For this review, use the dimensioned drawing (mm, ordinates from the lowest corner) and the shaded views. A direction names the side the tool comes from. Coordinates: 2 decimals unless noted, no trailing zeros. Loops run counter-clockwise (first coordinate to the right, second up) from the corner with the lowest first, then second, coordinate; pieces in that order, holes last. Notation, with made-up numbers: (-32, 59) -> (3, 59) arc R17 cw to (3, 75) -> close; hole circle Ø1 at (-6, 47.25). An arc over 180 degrees is marked (long way). Answer as a JSON object with one key per item and string values.
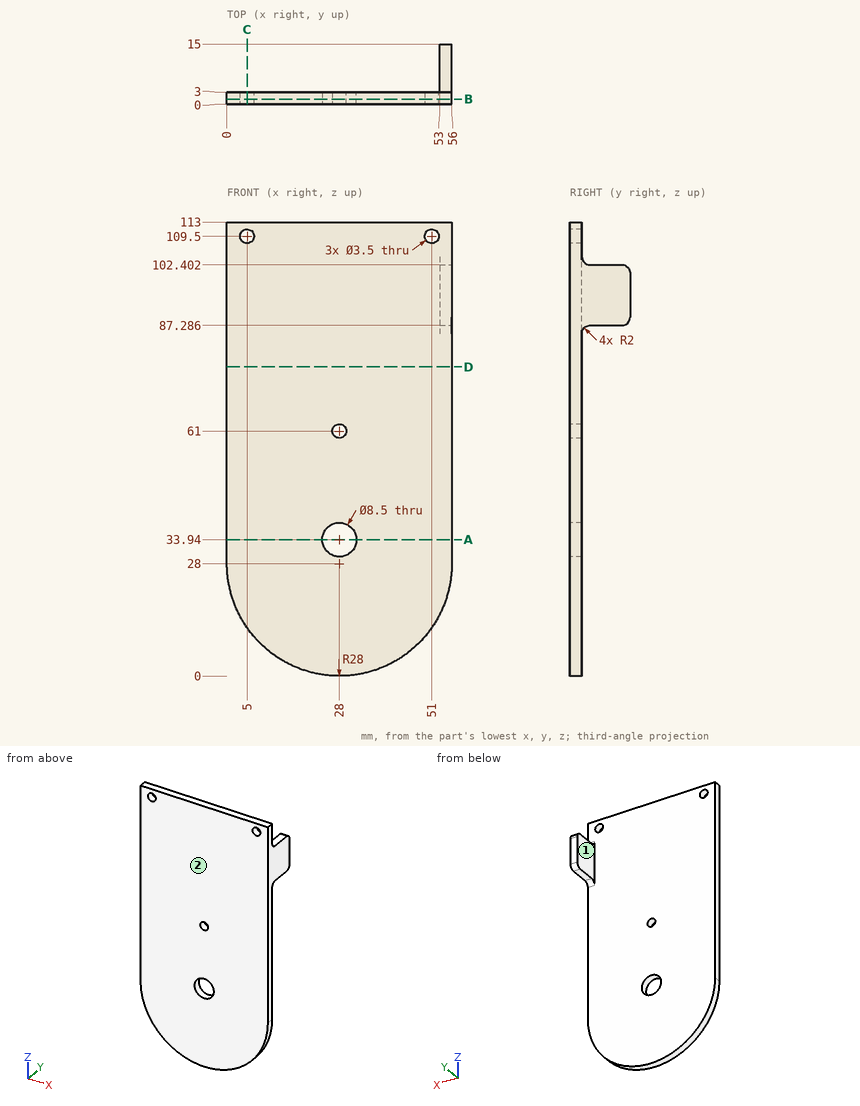
1) Wall thickness on probe 1 along Z at (x, y) = (28, 1.55); probe 2 along Y at (x, z) = (34.5, 76); probe 3 along Z at (x, y) = (5, 2.05): over which ranges is each line inside the solid? List them lowest first.
Completed:
{"probe 1": "0 to 29.69, 38.19 to 59.25, 62.75 to 113", "probe 2": "0 to 3", "probe 3": "12.03 to 107.75, 111.25 to 113"}
2) Add section B-B, the plane y = 1.25. Give the boundary of the cut face in (x, z), and give its area (3 significant figures).
Completed:
{"outline": "(0, 28) arc R28 ccw to (56, 28) -> (56, 113) -> (0, 113) -> close; hole circle Ø3.5 at (5, 109.5); hole circle Ø8.5 at (28, 33.94); hole circle Ø3.5 at (28, 61); hole circle Ø3.5 at (51, 109.5)", "area": "5,910 mm²"}
3) Clearance check with flat-ended pins moving along their axes: pin 1 Ø3 at (x, z) = (5, 109.5) entering from +Y; pin 2 Ø5 at (x, z) = (8.5, 62) entering from +Y; pin 3 Ø1 at (x, z) = (35, 73) entering from -Y; pin 4 Ø3.5 at (x, y) = (54.5, 8.5) entering from -Z. State where each tip first meets the part, or that it passes through.
Completed:
{"pin 1": "through", "pin 2": "y = 3", "pin 3": "y = 0", "pin 4": "z = 87.29"}
4) For the marked faces 1 and 2, list the 3-axis set-ups (+Z, -Z, +X, -X, +Y, -Y) from which the entire face can be reached by the end or side of a thin tool; tool diameter is ignored.
Completed:
{"face 1": "+Z, -Z, -X, +Y", "face 2": "+Z, -Z, +X, -X, -Y"}
5) Add section C-C, the plane x = 5. Give the boundary of the cut face in (y, z).
Completed:
{"outline": "(0, 12.03) -> (3, 12.03) -> (3, 107.75) -> (0, 107.75) -> close; (0, 111.25) -> (3, 111.25) -> (3, 113) -> (0, 113) -> close"}
6) Add section A-A, the plane z = 33.94. Give the boundary of the cut face in (x, y).
Completed:
{"outline": "(0, 0) -> (23.75, 0) -> (23.75, 3) -> (0, 3) -> close; (32.25, 0) -> (56, 0) -> (56, 3) -> (32.25, 3) -> close"}
7) Add section D-D, the plane z = 77. Give the boundary of the cut face in (x, y).
Completed:
{"outline": "(0, 0) -> (56, 0) -> (56, 3) -> (0, 3) -> close"}
